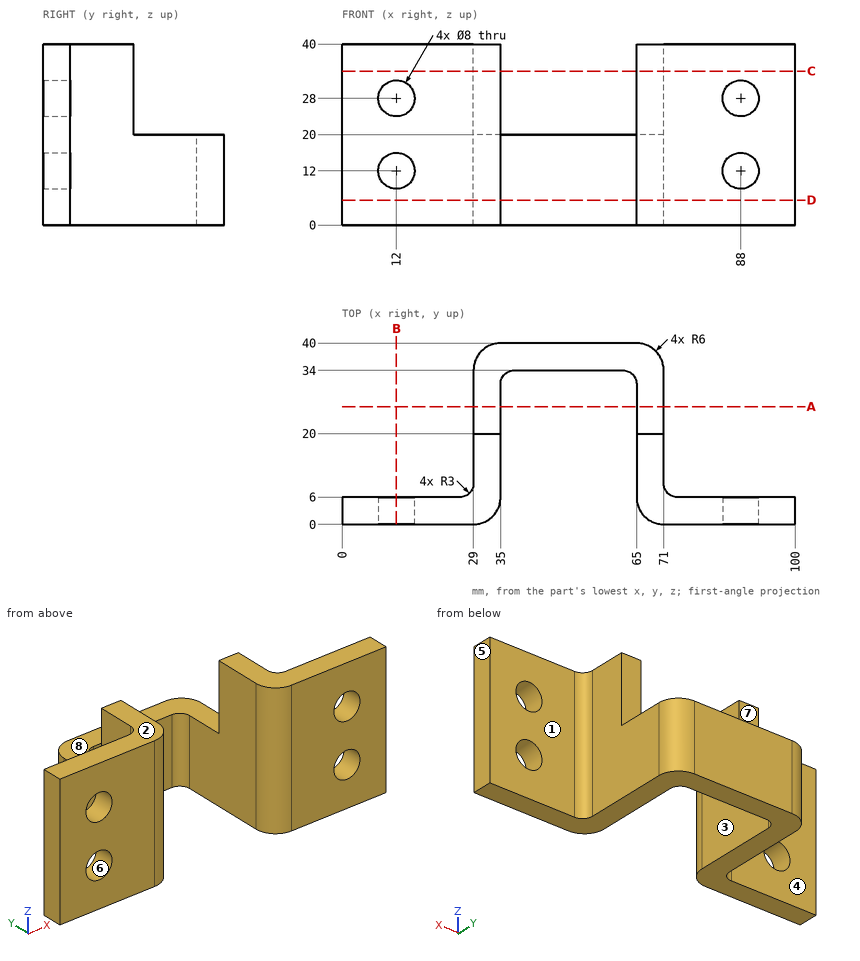
Input: dimensioned drawing with shaded views. Units: mm. Origin: part minimum x, y, z. A direction names the side the tool comes from. Round coordinates to 2 decimals unless told otherwise and drop trailing zeros. Write each loop counter-clockwise with the first axis right and the second up, starting at its lowest first coordinate (ties: lowest second). Pieces come first, ordered by that corner, then holes. Notation, with made-up numbers: (88, 38) - (141, 38) arc R33 ccw to (141, 70) - close; hole circle Ø6 at (-3.5, 12). An arc over 180 degrees is marked (long way). Write item = value, one per line.
(1) Section query C-C on z = 34. Output: boundary loops of the cut face in (x, y).
Geometry check:
outline = (0, 0) - (29, 0) arc R6 ccw to (35, 6) - (35, 20) - (29, 20) - (29, 9) arc R3 cw to (26, 6) - (0, 6) - close; (65, 6) arc R6 ccw to (71, 0) - (100, 0) - (100, 6) - (74, 6) arc R3 cw to (71, 9) - (71, 20) - (65, 20) - close
(2) Section query D-D on z = 5.5. Output: boundary loops of the cut face in (x, y).
Geometry check:
outline = (0, 0) - (29, 0) arc R6 ccw to (35, 6) - (35, 31) arc R3 cw to (38, 34) - (62, 34) arc R3 cw to (65, 31) - (65, 6) arc R6 ccw to (71, 0) - (100, 0) - (100, 6) - (74, 6) arc R3 cw to (71, 9) - (71, 34) arc R6 ccw to (65, 40) - (35, 40) arc R6 ccw to (29, 34) - (29, 9) arc R3 cw to (26, 6) - (0, 6) - close
(3) Section query A-A on y = 26. Output: boundary loops of the cut face in (x, z), then the cut area to 3 significant figures.
Geometry check:
outline = (29, 0) - (35, 0) - (35, 20) - (29, 20) - close; (65, 0) - (71, 0) - (71, 20) - (65, 20) - close
area = 240 mm^2
(4) Material intervals for probe 1 along Z at (x, y) = (88, 3); probe 2 along Y at (x, z) = (44.5, 10); probe 3 along Y at (x, z) = (82.5, 25), sorted ascending.
Geometry check:
probe_1 = 0 to 8, 16 to 24, 32 to 40
probe_2 = 34 to 40
probe_3 = 0 to 6
(5) Access query for the marked faces 1, 2, 3, 4 and 5. Directions: +Z, -Z, +X, -X, +Y, -Y. A direction counts if a zero-diameter tool reaches every point of the face in a straight line with its end or side. Return the directions, or none.
Geometry check:
face_1 = +Z, -Z, +X, +Y
face_2 = +Z, +X, -X, +Y, -Y
face_3 = +Z, -Z, -Y
face_4 = +Z, -Z, -X, +Y
face_5 = +Z, -Z, +X, +Y, -Y
(6) Section query B-B on x = 12. Output: boundary loops of the cut face in (y, z), then the cut area to 3 significant figures.
Geometry check:
outline = (0, 0) - (6, 0) - (6, 8) - (0, 8) - close; (0, 16) - (6, 16) - (6, 24) - (0, 24) - close; (0, 32) - (6, 32) - (6, 40) - (0, 40) - close
area = 144 mm^2
(7) Contact query for flat-ended pins moving along their axis: pin 1 Ø12.5 at (y, z) = (18.5, 12) entering from +X; pin 2 Ø9 at (x, z) = (88, 12) entering from -Y; pin 3 Ø1.8 at (x, z) = (66.5, 30.5) entering from +Y; pin 4 Ø5 at (x, y) = (27.5, 28) entering from +Z. Output: stop coordinate, or through.
Geometry check:
pin_1 = 71
pin_2 = 0
pin_3 = 20
pin_4 = 20
(8) Pull-direction query (Z, two-part tool) for the marked faces 6, 7 and 8; classes: +Z half, -Z half, draft (parallel to the pull), parting line (faces both ways), or undercut.
Geometry check:
face_6 = undercut
face_7 = draft
face_8 = +Z half
